Autodesk Inventor part; units mm, degrees
ref_plane "YZ Plane" through (0, 0, 0) normal (1, 0, 0) x (0, 1, 0)
ref_plane "XZ Plane" through (0, 0, 0) normal (0, 1, 0) x (-1, 0, 0)
ref_plane "XY Plane" through (0, 0, 0) normal (0, 0, 1) x (1, 0, 0)
sketch "스케치1" plane through (0, 0, 0) normal (0, 0, 1) x (1, 0, 0)
  arc A0 (0, 7) -> (0, -7) centre (0, 0) ccw
  arc A1 (0, 23) -> (0, -23) centre (0, 0) ccw
  line L0 (0, 0) -> (0, 23)
  line L1 (0, 0) -> (0, -23)
  dimension "d0" = 14
  dimension "d1" = 46
extrude "돌출1" add sketch "스케치1" along normal blind 4 contours A0 L1 A1 L0
sketch "스케치2" plane through (0, 0, 4) normal (0, 0, 1) x (1, 0, 0)
  arc A0 (0, 20) -> (0, -20) centre (0, 0) ccw
  arc A1 (0, 23) -> (0, -23) centre (0, 0) ccw
  line L0 (0, 20) -> (0, 29)
  line L1 (0, 0) -> (0, -29)
  arc A2 (-3, -28.8444) -> (0, -29) centre (0, 0) ccw
  arc A3 (0, 29) -> (-3, 28.8444) centre (0, 0) ccw
  line L2 (-3, 28.8444) -> (-3, 19.7737)
  line L3 (-3, -19.7737) -> (-3, -22.8035)
  line L4 (-3, -28.8444) -> (-3, -19.7737)
  line L5 (-3, 19.7737) -> (-3, 28.8444)
  line L6 (-3, 22.8035) -> (-3, 19.7737)
  line L7 (-3, -19.7737) -> (-3, -28.8444)
  line L8 (0, -29) -> (0, -20)
  line L9 (0, 20) -> (0, 29)
  line L10 (0, 29) -> (0, 20)
  line L11 (0, -20) -> (0, -29)
  dimension "d4" = 40
  dimension "d5" = 46
  dimension "d6" = 29
  dimension "d7" = 29
extrude "돌출2" add sketch "스케치2" along normal blind 12
sketch "스케치3" plane through (-3, -28.8444, 4) normal (-1, 0, 0) x (0, 0, 1)
  line L0 (0, 51.6479) -> (12, 51.6479)
  line L1 (12, 57.6888) -> (12, 51.6479)
  line L2 (0, 57.6888) -> (12, 57.6888)
  line L3 (0, 57.6888) -> (0, 51.6479)
  line L4 (12, 6.0409) -> (0, 6.0409)
  line L5 (0, 6.0409) -> (0, 0)
  line L6 (0, 0) -> (12, 0)
  line L7 (12, 6.0409) -> (12, 0)
  circle A0 centre (9, 3) radius 1.6
  circle A1 centre (3, 3) radius 1.6
  circle A2 centre (9, 54.6888) radius 1.6
  circle A3 centre (3, 54.6888) radius 1.6
  point P0 (-4, 28.8444)
  dimension "d16" = 3.2
  dimension "d17" = 3.2
  dimension "d18" = 3.2
  dimension "d19" = 3.2
  dimension "d20" = 3
  dimension "d21" = 3
  dimension "d22" = 3
  dimension "d23" = 3
  dimension "d24" = 3
  dimension "d25" = 3
  dimension "d26" = 3
  dimension "d27" = 3
extrude "돌출3" cut sketch "스케치3" against normal up to surface (3 mm away) contours A0 | A1 | A2 | A3
sketch "스케치5" plane through (0, 0, 16) normal (0, 0, 1) x (1, 0, 0)
  circle A0 centre (0, 0) radius 23
  arc A1 (-3, 22.8035) -> (-3, -22.8035) centre (0, 0) ccw
  line L0 (-23, 0) -> (-26, 0)
  line L1 (-23, 0) -> (-20, 0) construction
  line L2 (-26, 0) -> (-26, -3)
  line L3 (-26, -3) -> (-22.8035, -3)
  line L4 (-26, 0) -> (-26, 3)
  line L5 (-26, 0) -> (-23, 0) construction
  line L6 (-26, 3) -> (-22.8035, 3)
  dimension "d36" = 46
  dimension "d37" = 3
  dimension "d38" = 180
  dimension "d39" = 3
  dimension "d40" = 90
  dimension "d41" = 90
  dimension "d42" = 3
  dimension "d43" = 90
extrude "돌출5" add sketch "스케치5" against normal blind 16 contours A0 L0 L4 L6 | L3 L2 L0 A0
sketch "스케치6" plane through (-26, -3, 16) normal (-1, 0, 0) x (0, 0, 1)
  line L0 (0, 6) -> (0, 0)
  line L1 (0, 6) -> (-16, 6)
  line L2 (-16, 0) -> (-16, 6)
  line L3 (0, 0) -> (-16, 0)
  circle A0 centre (-3, 3) radius 1.25
  circle A1 centre (-9, 3) radius 1.25
  point P0 (-16, 3)
  dimension "d46" = 2.5
  dimension "d47" = 2.5
  dimension "d48" = 3
  dimension "d49" = 7
  dimension "d50" = 3
  dimension "d51" = 3
extrude "돌출6" cut sketch "스케치6" against normal blind 8 contours A0 | A1
sketch "스케치7" plane through (0, 0, 4) normal (0, 0, 1) x (1, 0, 0)
  circle A0 centre (0, 0) radius 13
  line L0 (0, 0) -> (-9.1924, 9.1924)
  line L1 (0, 0) -> (13, 0) construction
  line L2 (0, 0) -> (-9.1924, -9.1924)
  line L3 (0, 0) -> (13, 0) construction
  circle A1 centre (-9.1924, 9.1924) radius 1.6
  circle A2 centre (-9.1924, -9.1924) radius 1.6
  dimension "d54" = 26
  dimension "d55" = 135
  dimension "d56" = 135
  dimension "d57" = 3.2
  dimension "d58" = 3.2
extrude "돌출7" cut sketch "스케치7" against normal up to surface (4 mm away) contours A1 L0 A0 | A0 A1 | A2 A0 | A0 L2 A2 | L0 A1 A0 | A0 A2 L2
sketch "스케치8" plane through (0, 0, 0) normal (0, 0, -1) x (-1, 0, 0)
  arc A0 (3, 22.8035) -> (0, 23) centre (0, 0) ccw
  line L0 (3, 28.8444) -> (3, 22.8035)
  arc A1 (3, 28.8444) -> (0, 29) centre (0, 0) ccw
  line L1 (0, 23) -> (0, 29)
  arc A2 (0, -23) -> (3, -22.8035) centre (0, 0) ccw
  line L2 (0, -29) -> (0, -23)
  arc A3 (0, -29) -> (3, -28.8444) centre (0, 0) ccw
  line L3 (3, -22.8035) -> (3, -28.8444)
extrude "돌출8" add sketch "스케치8" against normal blind 4
properties part number "조인트4링크2고정부" material "알루미늄 6061"
Here's how the part is built. I have some questions about the finished solid (model axes, mm). A direction names the side the tool comes from. Round coordinates to 2 decimals unless told otherwise and drop trailing zeros. Order: outer loops, then holes, each group sorted by start corner. A loop starts at its lowest first (then second) coordinate and runs counter-clockwise, first axis right, second up. Notation, with made-up numbers: M 40.25,-4.75 L 74.25,-4.75 A25 cw 74.25,14.25 Z; hole C -37,52 d11. An arc over 180 degrees is marked long. Answer as CSV lines item,"result".
Item 1: Please list where these lines run through material, in increasing order: L1, parallel to Y at x = -8, z = 1; L2, parallel to Y at x = -1.5, z = 7; L3, parallel to Y at x = -2.1, z = 13. Write a range as [from, to].
From the geometry:
L1,"[-21.56, -10.26], [-8.13, 8.13], [10.26, 21.56]"
L2,"[-28.96, -27.44], [-24.24, -19.94], [19.94, 24.24], [27.44, 28.96]"
L3,"[-28.92, -27.44], [-24.24, -19.89], [19.89, 24.24], [27.44, 28.92]"
Item 2: Imagine slicing it at B-B on z = 13. List the corners of the cut face in (x, y) for me, and give its area (3 significant figures).
From the geometry:
outline,"M -26,-3 L -22.8,-3 A23 ccw -3,-22.8 L -3,-24.24 L 0,-24.24 L 0,-20 A20 cw -19.96,-1.25 L -26,-1.25 Z; M -26,1.25 L -19.96,1.25 A20 cw 0,20 L 0,24.24 L -3,24.24 L -3,22.8 A23 ccw -22.8,3 L -26,3 Z; M -3,-28.84 A29 ccw 0,-29 L 0,-27.44 L -3,-27.44 Z; M -3,27.44 L 0,27.44 L 0,29 A29 ccw -3,28.84 Z"
area,"223 mm2"
Item 3: For pin 1 (5 mm diameter, centred on x = -3, y = 1.5, fed in from -Z); pin 2 (1 mm diameter, centred on x = -23.5, z = 8, fed in from +Y); pin 3 (5 mm diameter, centred on x = -11, z = 2.5, fed in from -Y); pin 4 (3.5 mm diameter, centred on x = -9.19, y = 9.19, fed in from -Z), each with a flat end and sliding along its axis, tell me the tip position at first contact or that it passes through.
From the geometry:
pin 1,"through"
pin 2,"y = 3"
pin 3,"y = -21.37"
pin 4,"z = 0"
Item 4: Which directions (+Z, -Z, +X, -X, +Y, -Y) give clear straight access to the entire face, cutting with the end or side of a thin tool? Please do faces 1 (the cylindrical face through (-1.52, -26.82, 11.73)), 2 (the flat face through (-24, -3, 8)), 3 (the flat face through (-3, 28, 8)).
From the geometry:
face 1,"+X, -X"
face 2,"+Z, -Z, -X, -Y"
face 3,"+Z, -Z, -X, +Y"
Item 5: Imagine slicing it at D-D on z = 3. List the corners of the cut face in (x, y) for me.
From the geometry:
outline,"M -26,-3 L -22.8,-3 A23 ccw -3,-22.8 L -3,-28.84 A29 ccw 0,-29 L 0,-7 A7 cw 0,7 L 0,29 A29 ccw -3,28.84 L -3,22.8 A23 ccw -22.8,3 L -26,3 Z; hole C -9.19,-9.19 d3.2; hole C -9.19,9.19 d3.2"
Item 6: Imagine slicing it at C-C on x = -16.5. List the corners of the cut face in (y, z) for me.
From the geometry:
outline,"M -16.02,0 L 16.02,0 L 16.02,16 L 11.3,16 L 11.3,4 L -11.3,4 L -11.3,16 L -16.02,16 Z"
Item 7: We'd pull the mould along X, two halves only. Please class faces 4 (the cylindrical face through (-9.4, 10.78, 2.03)), 5 (the flat face through (-24, 3, 8)), 6 (the cylindrical face through (-16.412, 16.114, 7.888)): +X half, -X half, draft (parallel to the pull), parting line (faces both ways), or undercut.
From the geometry:
face 4,"undercut"
face 5,"draft"
face 6,"-X half"
Item 8: Imagine slicing it at A-A on y = 0. List the corners of the cut face in (x, z) for me, and give its area (3 significant figures).
From the geometry:
outline,"M -26,0 L -7,0 L -7,4 L -20,4 L -20,5.75 L -26,5.75 Z; M -26,8.25 L -20,8.25 L -20,11.75 L -26,11.75 Z; M -26,14.25 L -20,14.25 L -20,16 L -26,16 Z"
area,"118 mm2"
